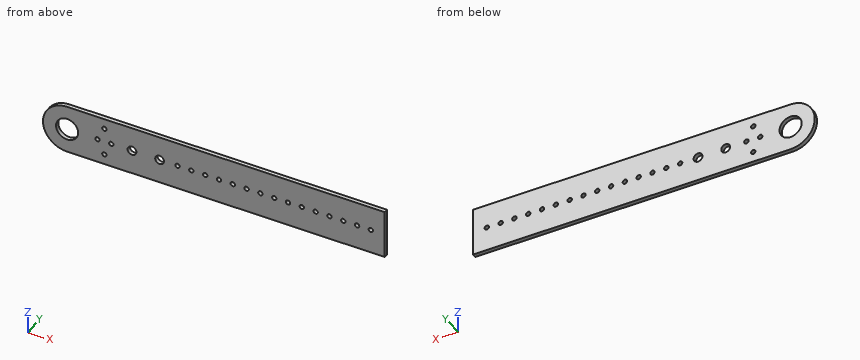
Autodesk Inventor part; units mm, degrees
ref_plane "YZ Plane" through (0, 0, 0) normal (1, 0, 0) x (0, 1, 0)
ref_plane "XZ Plane" through (0, 0, 0) normal (0, 1, 0) x (-1, 0, 0)
ref_plane "XY Plane" through (0, 0, 0) normal (0, 0, 1) x (1, 0, 0)
sketch "スケッチ1" plane through (0, 0, 0) normal (0, 1, 0) x (-1, 0, 0)
  line L0 (0, 0) -> (-230, 0)
  line L1 (-230, 0) -> (-230, -35)
  line L2 (-230, -35) -> (0, -35)
  line L3 (0, -35) -> (0, 0)
  arc A0 (0, -35) -> (0, 0) centre (0, -17.5) ccw
  dimension "d0" = 230
  dimension "d1" = 35
  dimension "d2" = 17.5
extrude "押し出し1" add sketch "スケッチ1" along normal blind 3
sketch "スケッチ2" plane through (0, 3, 0) normal (0, 1, 0) x (1, 0, 0)
  line L0 (0, 17.5) -> (238.6526, 17.5)
  line L1 (0, 0) -> (230, 0)
  arc A0 (0, 35) -> (0, 0) centre (0, 17.5) ccw
  point P0 (90, 17.5)
  point P1 (100, 17.5)
  point P2 (110, 17.5)
  point P3 (120, 17.5)
  point P4 (130, 17.5)
  point P5 (140, 17.5)
  point P6 (150, 17.5)
  point P7 (160, 17.5)
  point P8 (170, 17.5)
  point P9 (180, 17.5)
  point P10 (190, 17.5)
  point P11 (200, 17.5)
  point P12 (210, 17.5)
  point P13 (-17.5, 17.5)
  point P14 (220, 17.5)
  point P15 (80, 17.5)
  dimension "d5" = 17.5
  dimension "d13" = 10
  dimension "d14" = 10
  dimension "d15" = 10
  dimension "d16" = 10
  dimension "d17" = 10
  dimension "d18" = 10
  dimension "d19" = 10
  dimension "d20" = 10
  dimension "d21" = 10
  dimension "d22" = 10
  dimension "d23" = 10
  dimension "d24" = 10
  dimension "d35" = 17.5
  dimension "d67" = 10
  dimension "d78" = 10
  dimension "d96" = 80
hole "穴1" at (90, 3, -17.5) at (100, 3, -17.5) at (110, 3, -17.5) at (120, 3, -17.5) at (130, 3, -17.5) at (140, 3, -17.5) at (150, 3, -17.5) at (160, 3, -17.5) at (170, 3, -17.5) at (180, 3, -17.5) at (190, 3, -17.5) at (200, 3, -17.5) at (210, 3, -17.5) at (220, 3, -17.5) at (80, 3, -17.5) direction (0, -1, 0) diameter 3.2 end through all
sketch "スケッチ3" plane through (0, 3, 0) normal (0, 1, 0) x (1, 0, 0)
  line L0 (230, 35) -> (0, 35)
  point P0 (0, 0)
  point P1 (0, 17.5)
  dimension "d36" = 17.5
hole "穴2" at (0, 3, -17.5) direction (0, -1, 0) diameter 16 end through all
sketch "スケッチ4" plane through (0, 3, 0) normal (0, 1, 0) x (1, 0, 0)
  circle A0 centre (0, 17.5) radius 6
  circle A1 centre (0, 17.5) radius 8
  line L0 (-0.1439, 17.5) -> (-6.5454, 17.5)
  line L1 (-6.5454, 17.5) -> (7.5104, 17.5)
  point P0 (0, 0)
  point P1 (0, 11.5)
  point P2 (6, 17.5)
  point P3 (0, 23.5)
  point P4 (-6, 17.5)
  dimension "d44" = 12
  dimension "d45" = 0
hole "穴3" [suppressed]
sketch "スケッチ5" plane through (0, 3, 0) normal (0, 1, 0) x (1, 0, 0)
  circle A0 centre (0, 17.5) radius 8
  point P0 (0, 0)
  point P1 (15.8, 7)
  point P2 (15.8, 28)
  point P3 (24.9999, 17.5)
  dimension "d53" = 10.5
  dimension "d55" = 15.8
  dimension "d56" = 15.8
  dimension "d83" = 10.5
hole "穴4" [suppressed]
sketch "スケッチ6" plane through (0, 3, 0) normal (0, 1, 0) x (1, 0, 0)
  circle A0 centre (0, 17.5) radius 8 construction
  line L0 (0, 17.5) -> (230, 17.5) construction
  line L1 (230, 0) -> (230, 35) construction
  point P0 (0, 0)
  point P1 (67, 17.5)
  point P2 (47, 17.5)
  dimension "d69" = 47
  dimension "d70" = 20
hole "穴5" at (67, 3, -17.5) at (47, 3, -17.5) direction (0, -1, 0) diameter 6.4 end through all
sketch "スケッチ7" plane through (0, 3, 0) normal (0, 1, 0) x (1, 0, 0)
  circle A0 centre (0, 17.5) radius 8 construction
  circle A1 centre (0, 17.5) radius 12.5 construction
  point P0 (0, 0)
  point P1 (0, 5)
  point P2 (12.5, 17.5)
  point P3 (0, 30)
  point P4 (-12.5, 17.5)
  dimension "d84" = 25
  dimension "d87" = 360
hole "穴6" [suppressed]
sketch "スケッチ8" plane through (0, 3, 0) normal (0, 1, 0) x (1, 0, 0)
  line L0 (230, 0) -> (230, 35) construction
  line L1 (230, 17.5) -> (-17.5, 17.5) construction
  arc A0 (0, 35) -> (0, 0) centre (0, 17.5) ccw construction
  circle A1 centre (47, 17.5) radius 3.2 construction
  line L2 (27, 0) -> (27, 35) construction
  point P0 (32, 17.5)
  point P1 (22, 17.5)
  point P2 (27, 7.5)
  point P3 (27, 27.5)
  dimension "d97" = 15
  dimension "d98" = 10
  dimension "d106" = 5
  dimension "d107" = 10
  dimension "d108" = 10
hole "穴7" at (32, 3, -17.5) at (22, 3, -17.5) at (27, 3, -7.5) at (27, 3, -27.5) direction (0, -1, 0) diameter 3.2 end through all
properties part number "shoulder2_lower_right_plate" material "アルミニウム 5052"
The model under review builds one solid part; all positions refer to its coordinate system, in mm. Give positions to 0.01 mm unless a question says otherwise; leave off trailing zeros. Write each loop counter-clockwise with the first axis right and the second up, starting at its lowest first coordinate (ties: lowest second). Pieces come first, ordered by that corner, then holes.
(1) Consider section B-B, the plane z = -31.5. Give the boundary of the cut face in (x, y).
(2) To check wall thickness, follow L1, parallel to Z at x = 27, y = 1.3; L2, parallel to Z at x = 100, y = 0.6; L3, parallel to X at y = 1.65, z = -22.5 (1 decimal). State the ranges of each line that lie inside material, in increasing order.
(3) For P1, Ø1.9, axis at x = 130, z = -17.5, coming from the +Y side, flat-tipped, find the tip position at first contact; note if it passes through.
(4) Consider section A-A, the plane y = 0.85. Give the number of separate pieces and of enclosed holes in the cut face, and give its area (3 significant figures).
Returned:
1. outline: (-10.5, 0) - (230, 0) - (230, 3) - (-10.5, 3) - close
2. L1: z = -35 to -29.1, -25.9 to -9.1, -5.9 to 0
2. L2: z = -35 to -19.1, -15.9 to 0
2. L3: x = -16.8 to -6.2, 6.2 to 230
3. P1: passes through
4. separate pieces: 1
4. enclosed holes: 22
4. area: 8,110 mm2
